Can you work these out from the model? Positions are in its coordinate system, mm. Face numbers are marked on the shaded views. A direction names the side the tool comes from. Round coordinates to 2 decimals unless told otherwise and drop trailing zeros. Loops run counter-clockwise (first coordinate to the right, second up) from the corner with the lowest first, then second, coordinate; pieces in that order, holes last. Notation, with made-up numbers: M 15,-38.5 L 71,-38.5 A30 cw 71,-10.5 Z; hole C 48,52 d4. An arc over 180 degrees is marked long. Return JSON: item names as keys, results as strings.
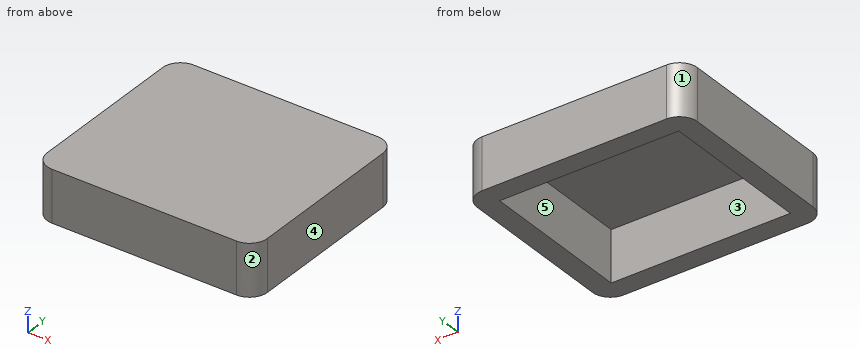
```python
from build123d import *

# Parameters (mm, degrees)
SKETCH1_W           = 350
SKETCH1_H           = 300
BOSS_EXTRUDE1_DEPTH = 100
BOSS_EXTRUDE2_DEPTH = 1


with BuildPart() as part:
    # Sketch1 → Boss-Extrude1 (new body)
    with BuildSketch(Plane.XY):
        with BuildLine():
            Line((-355, 340), (5, 340))
            ThreePointArc((5, 340), (29.748737342, 329.748737342), (40, 305))
            Line((40, 305), (40, -5))
            ThreePointArc((40, -5), (29.748737342, -29.748737342), (5, -40))
            Line((5, -40), (-355, -40))
            ThreePointArc((-355, -40), (-379.748737342, -29.748737342), (-390, -5))
            Line((-390, -5), (-390, 305))
            ThreePointArc((-390, 305), (-379.748737342, 329.748737342), (-355, 340))
        make_face()
        with Locations((-175, 150)):
            Rectangle(SKETCH1_W, SKETCH1_H, mode=Mode.SUBTRACT)
    extrude(amount=BOSS_EXTRUDE1_DEPTH)

    # Sketch2 → Boss-Extrude2 (add)
    with BuildSketch(Plane.XY.offset(100)):
        with BuildLine():
            Line((-355, -40), (5, -40))
            ThreePointArc((5, -40), (29.748737342, -29.748737342), (40, -5))
            Line((40, -5), (40, 305))
            ThreePointArc((40, 305), (29.748737342, 329.748737342), (5, 340))
            Line((5, 340), (-355, 340))
            ThreePointArc((-355, 340), (-379.748737342, 329.748737342), (-390, 305))
            Line((-390, 305), (-390, -5))
            ThreePointArc((-390, -5), (-379.748737342, -29.748737342), (-355, -40))
        make_face()
    extrude(amount=BOSS_EXTRUDE2_DEPTH)


solid = part.part
```
Q1. Suppose I cut it at C-C, the plane x = -295. Please give me the cut outline in (y, z).
Results:
{"outline": "M -40,0 L 0,0 L 0,100 L 300,100 L 300,0 L 340,0 L 340,101 L -40,101 Z"}
Q2. If I drill on line 1 along X through (y, z) = (225, 29); line 2 along Y through (x, z) = (-340, 46); line 3 along Z through (x, y) = (-152, 152), over which ranges is the centre line in solid material (lowest first)?
Results:
{"line 1": "x = -390 to -350, 0 to 40", "line 2": "y = -40 to 0, 300 to 340", "line 3": "z = 100 to 101"}
Q3. On a 3-axis mill with a long thin cutter (end or side, diameter ignored), from which of +Z, -Z, +X, -X, +Y, -Y can I reach the whole of each face in a straight line? I mean the marked faces 4 and 5. Say none if no direction works.
Results:
{"face 4": "+Z, -Z, +X, +Y, -Y", "face 5": "-Z"}
Q4. I'm going to push a flat-ended pin straight in: pin 1 Ø6 at (x, y) = (-291, 130) entering from -Z. Where does the tip first touch, or does it pass through?
Results:
{"pin 1": "stops at z = 100"}
Q5. Thinking about a two-plate mould opening in Y: for the marked faces 1, 2 and 3, which applies, pulls with the +Y half, pulls with the -Y half, needs draft (parallel to the pull), parting line crosses it, or undercut?
Results:
{"face 1": "pulls with the +Y half", "face 2": "pulls with the -Y half", "face 3": "undercut"}
Q6. Suppose I cut it at B-B, the plane y = 165. Please give me the cut outline in (x, z).
Results:
{"outline": "M -390,0 L -350,0 L -350,100 L 0,100 L 0,0 L 40,0 L 40,101 L -390,101 Z"}
Q7. Suppose I cut it at A-A, the plane z = 76. Please give me the cut outline in (x, y), plus the area to 3 significant figures.
Results:
{"outline": "M -390,-5 A35 ccw -355,-40 L 5,-40 A35 ccw 40,-5 L 40,305 A35 ccw 5,340 L -355,340 A35 ccw -390,305 Z; hole M -350,0 L 0,0 L 0,300 L -350,300 Z", "area": "57,300 mm2"}
